Read the model definition and answer for the solid it produces. Units are mm, in the model's axes. Coordinates: 2 decimals unless noted, no trailing zeros. Write each loop counter-clockwise with the first axis right and the second up, starting at its lowest first coordinate (ties: lowest second). Pieces come first, ordered by that corner, then holes.
(1) Section B-B on x = 0 is taken. Write down the section's boundary in (y, z).
(2) Section A-A on z = 0 is taken. Write down the section's boundary in (x, y).
(3) Section C-C on y = 1.5 is taken. Write down the section's boundary in (x, z).
(4) Find the intervals of material crossed by probe 1 along X at (y, z) = (1, 0); probe 2 along X at (y, z) = (4.5, 0); probe 3 along Y at (x, z) = (51, 31.5), in increasing order.
(5) Given pin 1 (1 mm diameter, centred on x = 46.5, y = 6.5, fed in from +Z); pin 2 (3 mm diameter, centred on y = 4, z = 4, fed in from +X), each flat-ended and moving along its own axis, determine where each tip first touches the part or whether it passes through.
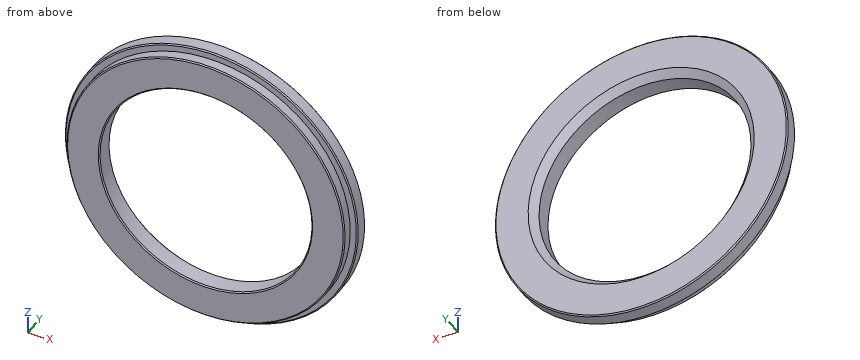
from build123d import *

# Parameters (mm, degrees)
CHANFRO1_SIZE = 3
CHANFRO2_SIZE = 0.5


with BuildPart() as part:
    # Esboço1 → Revolução1 (revolve)
    with BuildSketch(Plane.XY, mode=Mode.PRIVATE) as revolu_o1_sk:
        Polygon((45.25, 9.444130676), (62.5, 9.444130676), (62.5, 3.444130676), (59.356423034, 3.444130676), (59.356423034, -1.055869324), (45.25, -1.055869324), align=None)
    revolve(revolu_o1_sk.sketch.rotate(Axis((0, -46.025193798, 0), (0, 1, 0)), 90), axis=Axis((0, -46.025193798, 0), (0, 1, 0)))

    # Chanfro1
    chanfro1_edges = [part.edges().sort_by_distance(p)[0] for p in [
        (0, 9.444130676, 45.25),
    ]]
    chamfer(chanfro1_edges, length=CHANFRO1_SIZE)

    # Chanfro2
    chanfro2_edges = [part.edges().sort_by_distance(p)[0] for p in [
        (0, -1.055869324, 45.25),
        (0, -1.055869324, 59.356423034),
        (0, 3.444130676, 62.5),
        (0, 9.444130676, 62.5),
    ]]
    chamfer(chanfro2_edges, length=CHANFRO2_SIZE)


solid = part.part
Response:
1. outline: (-1.06, -58.86) - (-0.56, -59.36) - (3.44, -59.36) - (3.44, -62) - (3.94, -62.5) - (8.94, -62.5) - (9.44, -62) - (9.44, -48.25) - (6.44, -45.25) - (-0.56, -45.25) - (-1.06, -45.75) - close; (-1.06, 45.75) - (-0.56, 45.25) - (6.44, 45.25) - (9.44, 48.25) - (9.44, 62) - (8.94, 62.5) - (3.94, 62.5) - (3.44, 62) - (3.44, 59.36) - (-0.56, 59.36) - (-1.06, 58.86) - close
2. outline: (-62.5, 3.94) - (-62, 3.44) - (-59.36, 3.44) - (-59.36, -0.56) - (-58.86, -1.06) - (-45.75, -1.06) - (-45.25, -0.56) - (-45.25, 6.44) - (-48.25, 9.44) - (-62, 9.44) - (-62.5, 8.94) - close; (45.25, -0.56) - (45.75, -1.06) - (58.86, -1.06) - (59.36, -0.56) - (59.36, 3.44) - (62, 3.44) - (62.5, 3.94) - (62.5, 8.94) - (62, 9.44) - (48.25, 9.44) - (45.25, 6.44) - close
3. outline: circle Ø118.71 at (0, 0); hole circle Ø90.5 at (0, 0)
4. probe 1: x = -59.36 to -45.25, 45.25 to 59.36
4. probe 2: x = -62.5 to -45.25, 45.25 to 62.5
4. probe 3: y = 3.44 to 9.44
5. pin 1: stops at z = 42.31
5. pin 2: stops at x = 62.45
